Design review of the part built by this model. Coordinates are the model's own, in mm. Coordinates: 2 decimals unless noted, no trailing zeros. Order: outer loops, then holes, each group sorted by start corner. A loop starts at its lowest first (then second) coordinate and runs counter-clockwise, first axis right, second up. Notation, with made-up numbers: (-34.5, -36) -> (3.5, -36) arc R22 cw to (3.5, -20) -> close; hole circle Ø3 at (29, 64.25). An arc over 180 degrees is marked (long way). Write item = value, one per line.
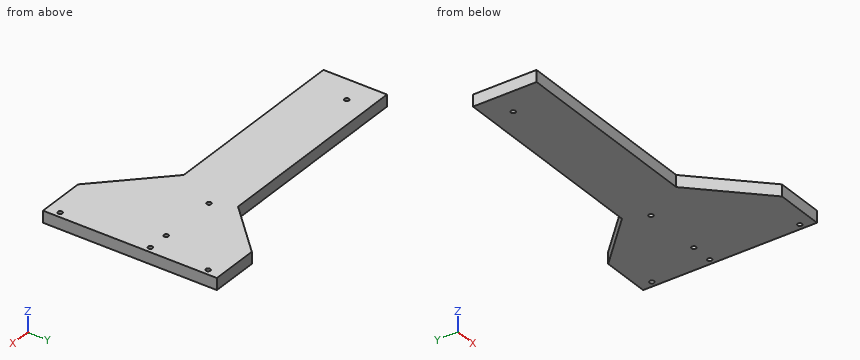
Autodesk Fusion 360 part; units mm, degrees
sketch "Top" plane through (0, 0, 0) normal (0, 0, 1) x (1, 0, 0)
  line L0 (145, 175) -> (220, 175)
  line L1 (220, 175) -> (220, -93)
  line L2 (220, -93) -> (145, -93)
  line L3 (-250, 2) -> (-250, 100)
  line L4 (145, 175) -> (70, 100)
  line L5 (145, -93) -> (50, 2)
  line L6 (70, 100) -> (-250, 100)
  line L7 (50, 2) -> (-250, 2)
  line L8 (211, 175) -> (211, -93) construction
  line L9 (220, 66) -> (-250, 66) construction
  circle A0 centre (211, 66) radius 3.5
  circle A1 centre (211, 155) radius 3.5
  circle A2 centre (211, -73) radius 3.5
  circle A3 centre (85, 66) radius 3.5
  circle A4 centre (-211, 66) radius 3.5
  circle A5 centre (177, 66) radius 3.5
  dimension "d3" = 75
  dimension "d4" = 75
  dimension "d5" = 95
  dimension "d6" = 95
  dimension "d7" = 268
  dimension "d8" = 470
  dimension "d9" = 75
  dimension "d10" = 9
  dimension "d11" = 34
  dimension "d12" = 7
  dimension "d13" = 7
  dimension "d14" = 7
  dimension "d15" = 89
  dimension "d16" = 139
  dimension "d17" = 7
  dimension "d18" = 7
  dimension "d19" = 7
  dimension "d20" = 34
  dimension "d21" = 92
  dimension "d22" = 296
extrude "Extrude1" add sketch "Top" along normal blind 18
(1) We need section A-A (z = 6). Write out the cut boundary in (x, y), and give its area (3 significant figures).
Report:
outline = (-250, 2) -> (50, 2) -> (145, -93) -> (220, -93) -> (220, 175) -> (145, 175) -> (70, 100) -> (-250, 100) -> close; hole circle Ø7 at (-211, 66); hole circle Ø7 at (85, 66); hole circle Ø7 at (177, 66); hole circle Ø7 at (211, -73); hole circle Ø7 at (211, 66); hole circle Ø7 at (211, 155)
area = 65,900 mm²
(2) We need section C-C (y = 110.5). Write out the cut boundary in (x, z).
Report:
outline = (80.5, 0) -> (220, 0) -> (220, 18) -> (80.5, 18) -> close
(3) We need section B-B (x = 124). Write out the cut boundary in (y, z), and give its area (3 significant figures).
Report:
outline = (-72, 0) -> (154, 0) -> (154, 18) -> (-72, 18) -> close
area = 4,070 mm²
(4) Insertion check: pin 1 (6 mm diameter, centred on x = -51.5, z = 6.5, fed in from +Y); pin 2 (8 mm diameter, centred on x = 211, y = 66, fed in from +Z); pin 3 (4 mm diameter, centred on x = -13, z = 5, fed in from -Y); pin 4 (4 mm diameter, centred on x = 80, z = 11.5, fed in from -Y). Each pin has a flat end and moves straight along its axis. Give the tip position at first contact, or say it passes through.
Report:
pin_1 = 100
pin_2 = 18
pin_3 = 2
pin_4 = -30
(5) For L1, parallel to Y at x = 211, z = 12; L2, parallel to Y at x = 177, z = 4.5; L3, parallel to Y at x = -125, z = 8.25, list the stretches that pass through material, from the lowest coordinate up.
Report:
L1 = -93 to -76.5, -69.5 to 62.5, 69.5 to 151.5, 158.5 to 175
L2 = -93 to 62.5, 69.5 to 175
L3 = 2 to 100
